Part print with two shaded views. Sizes in mm from the minimum x, y, z corner. A direction names the side the tool comes from. Round coordinates to 2 decimals unless told otherwise and drop trailing zeros. Order: outer loops, then holes, each group sorted by start corner. A loop starts at its lowest first (then second) coordinate and runs counter-clockwise, first axis right, second up. Notation, with made-up numbers: (-16.5, 51) - (-10.5, 51) arc R18 ccw to (-10.5, 83) - close; hole circle Ø1 at (84, -2.5). An arc over 180 degrees is marked (long way). Use one line per item in the form item = value.
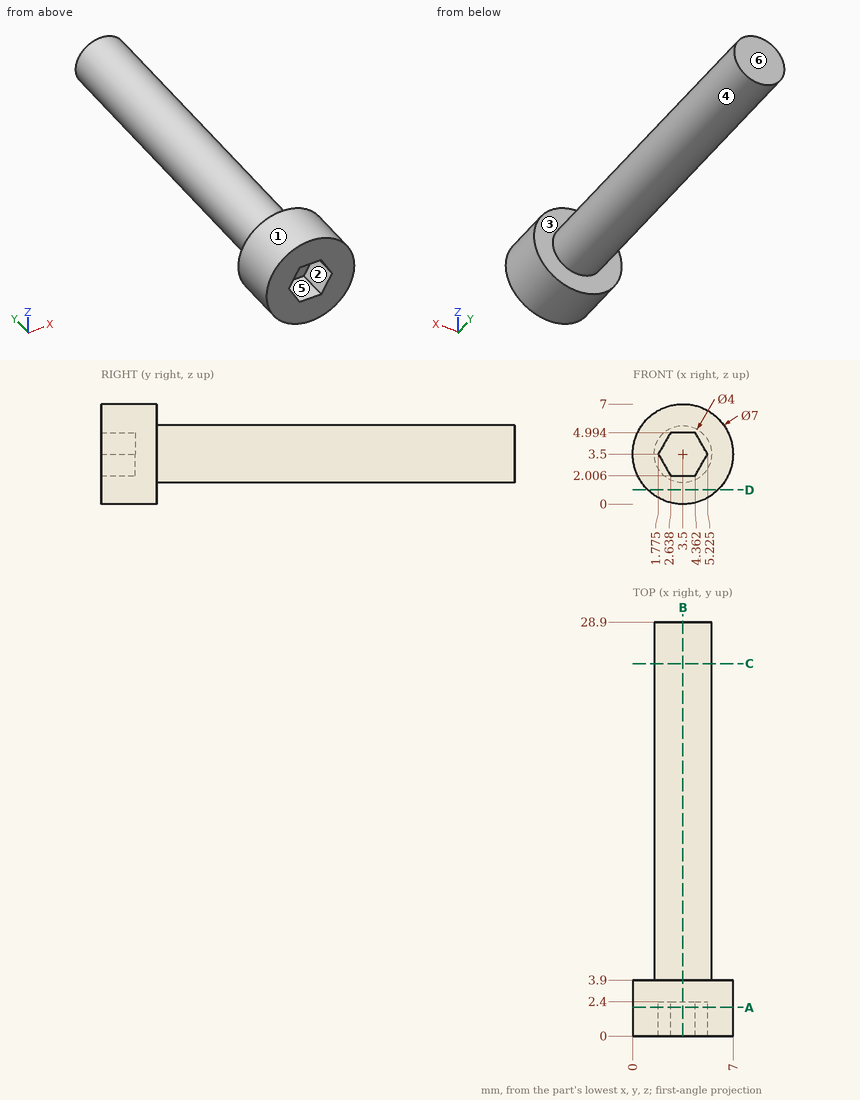
(1) Slice it at D-D on z = 1. Give the cut face in (x, y), then the cut area to 3 significant figures.
Report:
outline = (1.05, 0) - (5.95, 0) - (5.95, 3.9) - (1.05, 3.9) - close
area = 19.1 mm2
(2) Slice it at B-B on x = 3.5. Give the cut face in (y, z), then the cut area to 3 significant figures.
Report:
outline = (0, 0) - (3.9, 0) - (3.9, 1.5) - (28.9, 1.5) - (28.9, 5.5) - (3.9, 5.5) - (3.9, 7) - (0, 7) - (0, 4.99) - (2.4, 4.99) - (2.4, 2.01) - (0, 2.01) - close
area = 120 mm2
(3) Tool access for the marked faces 4, 5 and 6: list every direction of +Z, -Z, +X, -X, +Y, -Y with a clear straight run to the whole face (end or side of a thin tool).
Report:
face_4 = +Y
face_5 = -Y
face_6 = +Z, -Z, +X, -X, +Y
(4) Slice it at A-A on y = 2. Give the cut face in (x, z) (1 decimal).
Report:
outline = circle Ø7 at (3.5, 3.5); hole (1.8, 3.5) - (2.6, 2) - (4.4, 2) - (5.2, 3.5) - (4.4, 5) - (2.6, 5) - close
(5) Pin check, flat tips, straight feed: pin 1 (1 mm diameter, centred on y = 26, z = 1.5, fed in from -X) (1 decimal); pin 2 (1.5 mm diameter, centred on x = 3, z = 4, fed in from -Y); pin 3 (1.5 mm diameter, centred on y = 18.5, z = 6, fed in from -X) (1 decimal). Stop position of each tip, or through.
Report:
pin_1 = 2.2
pin_2 = 2.4
pin_3 = 2.5
(6) Pull direction Z, two halves, no side cores. Call the marked faces 1, 2 and 3: released by +Z, released by -Z, zero draft, split by the parting line, or undercut.
Report:
face_1 = split by the parting line
face_2 = undercut
face_3 = zero draft
(7) Probe probe 1 along Y at (x, z) = (6.5, 3); probe 2 along Y at (x, z) = (3.25, 3.5); probe 3 along X at (y, z) = (24.25, 3.5). List the from-to ranges inside material, lowest first. Write a range as [from, to].
Report:
probe_1 = [0, 3.9]
probe_2 = [2.4, 28.9]
probe_3 = [1.5, 5.5]
(8) Slice it at C-C on y = 26. Give the cut face in (x, z).
Report:
outline = circle Ø4 at (3.5, 3.5)
